```python
from build123d import *

# Parameters (mm, degrees)
F0_R     = 76.2
F1_DEPTH = 3.175
F2_R     = 50.8
F3_DEPTH = 63.5
F4_R     = 76.2
F5_DEPTH = 3.175
F6_R     = 12.7
F7_DEPTH = 254


with BuildPart() as f1:
    # F0 (on Front) → F1 (new body)
    with BuildSketch(Plane.XZ):
        Circle(F0_R)
    extrude(amount=F1_DEPTH)

    # F2 (on face) → F3 (join)
    with BuildSketch(Plane.XZ.offset(3.175)):
        Circle(F2_R)
    extrude(amount=F3_DEPTH)

    # F4 (on face) → F5 (join)
    with BuildSketch(Plane.XZ.offset(66.675)):
        Circle(F4_R)
    extrude(amount=F5_DEPTH)

    # F6 (on face) → F7 (cut)
    with BuildSketch(Plane.XZ.offset(69.85)):
        Circle(F6_R)
    extrude(amount=-F7_DEPTH, mode=Mode.SUBTRACT)


solid = f1.part
```
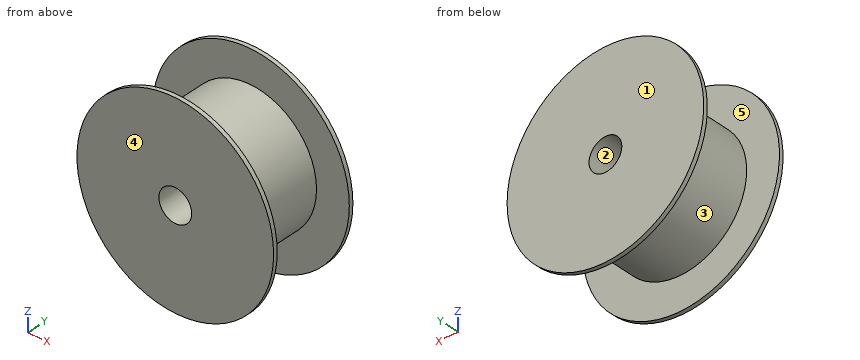
The listing builds one solid part. Answer for the finished solid, in the listing's coordinates (mm). Face numbers are marked on the shaded views. A direction names the side the tool comes from. Round coordinates to 2 decimals unless told otherwise and drop trailing zeros. Loops run counter-clockwise (first coordinate to the right, second up) from the corner with the lowest first, then second, coordinate; pieces in that order, holes last. Notation, with made-up numbers: (5, 45.5) - (62, 45.5) arc R17 cw to (62, 60.5) - close; hole circle Ø11 at (-33, 39.5). An arc over 180 degrees is marked (long way). Return JSON: item names as keys, results as strings. Group by question number.
1. The part is cut by section B-B on x = 0. Determine the outline of the cut face in (y, z) (3 decimals), then the cut area to 3 significant figures.
2. The part is cut by section A-A on z = 0. Determine the outline of the cut face in (x, y) (3 decimals), then the cut area to 3 significant figures.
3. The mould has two halves that part along Z. Classify the marked faces 1, 2 and 3: pulls with the +Z half, pulls with the -Z half, needs draft (parallel to the pull), parting line crosses it, or undercut.
4. Consider probe 1 along Y at (x, z) = (50.5, -16) (3 decimals); probe 2 along Z at (x, y) = (-1, -61); probe 3 along Z at (x, y) = (-14, -18.5). Determine where each line is inside the solid, lowest interval first.
5. Each of these flat-tipped pins is pushed along its axis until it touches: P1, Ø8, axis at y = -61, z = 17.5, coming from the -X side; P2, Ø3, axis at y = -53, z = 34, coming from the +X side; P3, Ø6, axis at y = -38, z = 15.5, coming from the -X side; P4, Ø8, axis at x = -1, z = 6, coming from the -Y side. Where does it stop, or does it pass through?
6. Which of the six approach directions +Z, -Z, +X, -X, +Y, -Y give full straight-line access (tool end or side, diameter ignored) to the marked faces 4 and 5?
7. The part is cut by section D-D on x = 63.5. Determine the outline of the cut face in (y, z) (3 decimals), then the cut area to 3 significant figures.
8. The part is cut by section C-C on y = -53. Determine the outline of the cut face in (x, z).
Resolved:
{
 "1": {"outline": "(-69.85, -76.2) - (-66.675, -76.2) - (-66.675, -50.8) - (-3.175, -50.8) - (-3.175, -76.2) - (0, -76.2) - (0, -12.7) - (-69.85, -12.7) - close; (-69.85, 12.7) - (0, 12.7) - (0, 76.2) - (-3.175, 76.2) - (-3.175, 50.8) - (-66.675, 50.8) - (-66.675, 76.2) - (-69.85, 76.2) - close", "area": "5,650 mm²"},
 "2": {"outline": "(-76.2, -69.85) - (-12.7, -69.85) - (-12.7, 0) - (-76.2, 0) - (-76.2, -3.175) - (-50.8, -3.175) - (-50.8, -66.675) - (-76.2, -66.675) - close; (12.7, -69.85) - (76.2, -69.85) - (76.2, -66.675) - (50.8, -66.675) - (50.8, -3.175) - (76.2, -3.175) - (76.2, 0) - (12.7, 0) - close", "area": "5,650 mm²"},
 "3": {"face 1": "needs draft", "face 2": "undercut", "face 3": "parting line crosses it"},
 "4": {"probe 1": "y = -69.85 to -66.675, -3.175 to 0", "probe 2": "z = -50.79 to -12.66, 12.66 to 50.79", "probe 3": "z = -48.83 to 48.83"},
 "5": {"P1": "stops at x = -48.97", "P2": "stops at x = 39.04", "P3": "stops at x = -49.24", "P4": "passes through"},
 "6": {"face 4": "+Z, -Z, +X, -X, -Y", "face 5": "none"},
 "7": {"outline": "(-69.85, -42.121) - (-66.675, -42.121) - (-66.675, 42.121) - (-69.85, 42.121) - close; (-3.175, -42.121) - (0, -42.121) - (0, 42.121) - (-3.175, 42.121) - close", "area": "535 mm²"},
 "8": {"outline": "circle Ø101.6 at (0, 0); hole circle Ø25.4 at (0, 0)"}
}
